Input: part model. Units: mm. Frame: model coordinates. Face numbers are marked on the shaded views. A direction names the side the tool comes from. Give positions to 0.01 mm unless a question says otherwise; leave off trailing zeros. Order: outer loops, then holes, each group sorted by start corner. A loop starts at its lowest first (then second) coordinate and runs counter-clockwise, first axis right, second up. Notation, with made-up numbers: (57, 83.5) - (65, 83.5) arc R35 cw to (65, 119.5) - close; hole circle Ø3 at (70, -2.5). An arc over 180 degrees is marked (long way). Use a Markdown table: item, result.
from build123d import *

# Parameters (mm, degrees)
F0_R           = 9.398
F1_DEPTH       = 19.05
F2_R           = 3.175
F3_DEPTH       = 3.175
F4_R           = 3.175
F5_DEPTH       = 3.175
F6_R           = 3.175
F7_DEPTH       = 127
F10_DEPTH      = 25.4
F11_DEPTH      = 25.4
F11_DEPTH_BACK = 25.4


# Not quite as in the source:
# - a feature of the source that left no trace in its solid (it failed there, or was rolled back) is left out


with BuildPart() as f1:
    # F0 (on Front) → F1 (new body)
    with BuildSketch(Plane.XZ):
        Circle(F0_R)
    extrude(amount=F1_DEPTH)

    # F2 (on face) → F3 (join)
    with BuildSketch(Plane.XZ.offset(19.05)):
        Circle(F2_R)
    extrude(amount=F3_DEPTH)

    # F4 (on face) → F5 (join)
    with BuildSketch(Plane(origin=(0, 0, 0), x_dir=(-1, 0, 0), z_dir=(0, 1, 0))):
        Circle(F4_R)
    extrude(amount=F5_DEPTH)

    # F6 (on Right) → F7 (cut)
    with BuildSketch(Plane.YZ):
        with Locations((-9.5303244889, 0)):
            Circle(F6_R)
    extrude(amount=-F7_DEPTH, mode=Mode.SUBTRACT)

    # F6 (on Right) → F10 (cut)
    with BuildSketch(Plane.YZ):
        with Locations((-9.5303244889, 0)):
            Circle(F6_R)
    extrude(amount=-F10_DEPTH, mode=Mode.SUBTRACT)

    # F6 (on Right) → F11 (cut, two sides)
    with BuildSketch(Plane.YZ) as f11_sk:
        with Locations((-9.5303244889, 0)):
            Circle(F6_R)
    extrude(amount=-F11_DEPTH, mode=Mode.SUBTRACT)
    extrude(f11_sk.sketch, amount=F11_DEPTH_BACK, mode=Mode.SUBTRACT)


solid = f1.part
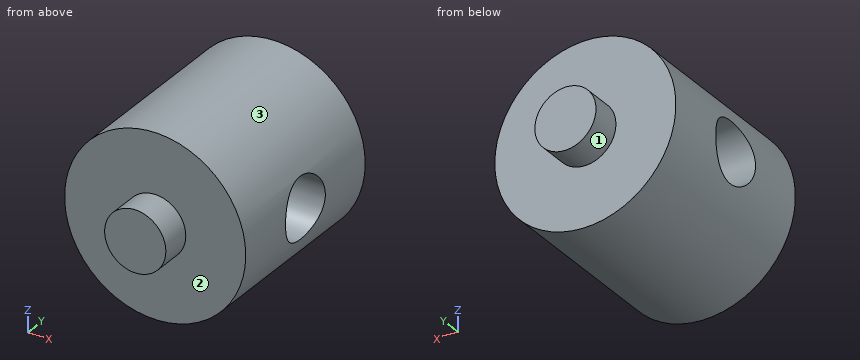
1. Section query B-B (x = -2.25). Return loops of the section in (y, z) (3 decimals), then the cut area to 3 significant figures.
Response:
| item | result |
|---|---|
| outline | (-22.225, -2.24) - (-19.05, -2.24) - (-19.05, -9.125) - (0, -9.125) - (0, -2.24) - (3.175, -2.24) - (3.175, 2.24) - (0, 2.24) - (0, 9.125) - (-19.05, 9.125) - (-19.05, 2.24) - (-22.225, 2.24) - close; hole circle Ø6.35 at (-9.53, 0) |
| area | 344 mm^2 |
2. Pin query (flat end, axial travel): pin 1 (6 mm diameter, centred on x = 7, y = -18, fed in from +Z); pin 2 (10 mm diameter, centred on x = -6.5, y = -7, fed in from -Z); pin 3 (1.5 mm diameter, centred on y = 0.5, z = -6.5, fed in from +X); pin 4 (7.5 mm diameter, centred on y = -9.53, z = 0, fed in from -X). Return the tip coordinate at first contact, or that it passes through.
Response:
| item | result |
|---|---|
| pin 1 | stops at z = 8.5 |
| pin 2 | stops at z = -9.28 |
| pin 3 | stops at x = 7.28 |
| pin 4 | stops at x = -9.4 |
3. Set-up query: the marked faces 1, 2 and 3. Return all of +Z, -Z, +X, -X, +Y, -Y with unobstructed straight access to the full face (end or side cutting, diameter ignored); none if empty.
Response:
| item | result |
|---|---|
| face 1 | +Y |
| face 2 | -Y |
| face 3 | +Y, -Y |
4. Section query C-C (y = -20.5). Return loops of the section in (x, z) (3 decimals).
Response:
| item | result |
|---|---|
| outline | circle Ø6.35 at (0, 0) |
5. Material intervals for line 1 along Y through (x, z) = (5.25, 0); line 2 along Y through (x, z) = (-2.5, 0) (3 decimals); line 3 along X through (y, z) = (-2, 0.25), sorted ascending.
Response:
| item | result |
|---|---|
| line 1 | y = -19.05 to -12.71, -6.36 to 0 |
| line 2 | y = -22.225 to -12.705, -6.355 to 3.175 |
| line 3 | x = -9.39 to 9.39 |
6. Section query D-D (y = -10.5). Return loops of the section in (x, z), then the cut area to 3 significant figures.
Response:
| item | result |
|---|---|
| outline | (-8.9, -3.02) arc R9.4 ccw to (8.9, -3.02) - close; (-8.9, 3.02) - (8.9, 3.02) arc R9.4 ccw to start |
| area | 166 mm^2 |
7. Section query A-A (z = 0). Return loops of the section in (x, y) (3 decimals).
Response:
| item | result |
|---|---|
| outline | (-9.398, -19.05) - (-3.175, -19.05) - (-3.175, -22.225) - (3.175, -22.225) - (3.175, -19.05) - (9.398, -19.05) - (9.398, -12.705) - (-9.398, -12.705) - close; (-9.398, -6.355) - (9.398, -6.355) - (9.398, 0) - (3.175, 0) - (3.175, 3.175) - (-3.175, 3.175) - (-3.175, 0) - (-9.398, 0) - close |
